The listing builds one solid part. Answer for the finished solid, in the listing's coordinates (mm). A direction names the side the tool comes from. Give positions to 0.01 mm unless a question says otherwise; leave off trailing zeros. Loops run counter-clockwise (first coordinate to the right, second up) from the corner with the lowest first, then second, coordinate; pieces in that order, holes last. Notation, with made-up numbers: M -33.75,22.5 L -10.75,22.5 A28 cw -10.75,54.5 Z; hole C 37,34.5 d1. An arc over 180 degrees is marked long. One line per item, written item: value. Start each with the question number.
Q1. Consider L1, parallel to Y at x = 0, z = -0.35 (3 decimals); L2, parallel to Y at x = 0, z = 7; L3, parallel to Z at x = -6, y = -18. Determine where each line is inside the solid, lowest interval first.
Q2. A cutting plane is placed at B-B, the plane z = 9.5. Determine the outline of the cut face in (x, y) (3 decimals), and give its area (3 significant figures).
Q3. A cutting plane is placed at A-A, the plane z = 14.25. Determine the outline of the cut face in (x, y).
Q4. The mould has two halves that part along Z. Classify faces 1 (the flat face through (20, 0, 15.367)), 2 (the flat face through (0, 13, 0.762)), 3 (the flat face through (-22, 0, 6.477)), 4 (the cylindrical face through (-0.99, 1.97, -1.17)): +Z half, -Z half, draft (parallel to the pull), parting line (faces both ways), or undercut.
Q5. For faces 5 (the flat face through (0, 21.59, -2)), 6 (the flat face through (-3, 0, 10.287)), 7 (the flat face through (0, -21.59, -2)), determine the directions among +Z, -Z, +X, -X, +Y, -Y from which every point of the face is accessible in a straight line to the end or side of a thin tool.
Q6. Flat-ended cylindrical pins translate along their axes: pin 1 (4 mm diameter, centred on y = 0.5, z = 12.5, fed in from -X); pin 2 (24.5 mm diameter, centred on x = 0, y = 9.525, fed in from +Z); pin 3 (4.5 mm diameter, centred on x = 1.5, y = 13, fed in from -Z). Find the tip coordinate at first contact, or state that the pin passes through.
from build123d import *

# Parameters (mm, degrees)
F0_W      = 43.18
F0_H      = 43.18
F3_DEPTH  = 3.048
F3_FACE_W = 43.18
F3_FACE_H = 43.18
F2_W      = 36.83
F2_H      = 36.83
F5_R      = 7.62
F6_DEPTH  = 3.81
F7_R      = 3.2639
F8_DEPTH  = 25.4
F9_W      = 36.83
F9_H      = 36.83
F9_W_2    = 43.18
F9_H_2    = 2.54
F9_R      = 3.2639
F10_DEPTH = 3.81
F11_W     = 3.81
F11_H     = 48.26
F12_DEPTH = 5.08


# Not quite as in the source:
# - a feature names something its author has since deleted; it is built from what else it names


with BuildPart() as f3:
    # F0 (on Top) → F3 (new body)
    with BuildSketch(Plane.XY):
        Rectangle(F0_W, F0_H)
    extrude(amount=-F3_DEPTH)

    # F3_face (on face) → F4 section 0
    with BuildSketch(Plane.XY):
        Rectangle(F3_FACE_W, F3_FACE_H)
    # F2 (on offset) → F4 section 1
    with BuildSketch(Plane.XY.offset(6.477)):
        with Locations((-0.127, -0.127)):
            Rectangle(F2_W, F2_H)
    loft()

    # F5 (on face) → F6 (cut)
    with BuildSketch(Plane(origin=(0, 0, -3.048), x_dir=(1, 0, 0), z_dir=(0, 0, -1))):
        with Locations((0, -9.525)):
            Circle(F5_R)
    extrude(amount=-F6_DEPTH, mode=Mode.SUBTRACT)

    # F7 (on face) → F8 (cut)
    with BuildSketch(Plane(origin=(0, 0, 0.762), x_dir=(1, 0, 0), z_dir=(0, 0, -1))):
        with Locations((0, -9.525)):
            Circle(F7_R)
    extrude(amount=-F8_DEPTH, mode=Mode.SUBTRACT)

    # F9 (on face) → F10 (join)
    with BuildSketch(Plane.XY.offset(6.477)):
        Polygon((-21.59, 24.13), (-21.59, 21.59), (-21.59, -21.59), (21.59, -21.59), (21.59, 21.59), (21.59, 24.13), align=None)
        with Locations((-0.127, -0.127)):
            Rectangle(F9_W, F9_H, mode=Mode.SUBTRACT)
        Polygon((-21.59, -21.59), (-21.59, 21.59), (-21.59, 24.13), (-24.13, 24.13), (-24.13, -24.13), (-21.59, -24.13), align=None)
        with Locations((0, -22.86)):
            Rectangle(F9_W_2, F9_H_2)
        with Locations((-0.127, -0.127)):
            Rectangle(F9_W, F9_H)
        with Locations((0, 9.525)):
            Circle(F9_R, mode=Mode.SUBTRACT)
    extrude(amount=F10_DEPTH)

    # F11 (on face) → F12 (join)
    with BuildSketch(Plane.XY.offset(10.287)):
        with Locations((19.685, 0)):
            Rectangle(F11_W, F11_H)
    extrude(amount=F12_DEPTH)


solid = f3.part
Answer block:
1. L1: -21.59 to 1.905, 17.145 to 21.59
1. L2: -24.13 to 6.26, 12.79 to 24.13
1. L3: -3.05 to 10.29
2. outline: M -24.13,-24.13 L 21.59,-24.13 L 21.59,24.13 L -24.13,24.13 Z; hole C 0,9.525 d6.528
2. area: 2,170 mm^2
3. outline: M 17.78,-24.13 L 21.59,-24.13 L 21.59,24.13 L 17.78,24.13 Z
4. face 1: +Z half
4. face 2: -Z half
4. face 3: undercut
4. face 4: draft
5. face 5: -Z, +X, -X, +Y
5. face 6: +Z, -X, +Y, -Y
5. face 7: -Z, +X, -X, -Y
6. pin 1: x = 17.78
6. pin 2: z = 10.29
6. pin 3: z = 0.76
